Autodesk Inventor part; units mm, degrees
ref_plane "YZ Plane" through (0, 0, 0) normal (1, 0, 0) x (0, 1, 0)
ref_plane "XZ Plane" through (0, 0, 0) normal (0, 1, 0) x (-1, 0, 0)
ref_plane "XY Plane" through (0, 0, 0) normal (0, 0, 1) x (1, 0, 0)
sketch "Sketch1" plane through (0, 0, 0) normal (0, 1, 0) x (-1, 0, 0)
  arc A0 (9.525, 0) -> (0, -9.525) centre (0, 0) ccw
  line L0 (0, 0) -> (0, -696.722) construction
  arc A1 (0, -687.197) -> (9.525, -696.722) centre (0, -696.722) ccw
  line L1 (9.525, -696.722) -> (9.525, 0)
  line L2 (-9.525, 0) -> (-9.525, -696.722)
  circle A2 centre (0, -696.722) radius 4.7625
  circle A3 centre (0, 0) radius 4.7625
  dimension "d0" = 19.05
  dimension "d2" = 19.05
  dimension "d3" = 9.525
  dimension "d4" = 9.525
  dimension "d10" = 696.722
extrude "Extrusion2" add sketch "Sketch1" along normal blind 6.35
properties part number "steeringlinkage" material "Steel, Mild"
Source: CAD feature listing. Evaluate the final solid. Frame: model axes, mm. Coordinates: 2 decimals unless noted, no trailing zeros. Write each question's results on one line, items separated by ' | '. Start each with the question number.
1. Material intervals for L1, parallel to Z at x = 0.5, y = 4.5; L2, parallel to Z at x = 0, y = 3.5 (1 decimal); L3, parallel to Z at x = -5.75, y = 3.25, sorted ascending.
2. Pin query (flat end, axial travel): pin 1 (2 mm diameter, centred on x = 4.5, y = 5.5, fed in from +Z); pin 2 (5.5 mm diameter, centred on x = 0, z = 0, fed in from +Y) (3 decimals). Return the tip coordinate at first contact, or that it passes through.
3. Section A-A, the plane x = 0. State how many separate pieces and enclosed holes the cut face has, then the cut area to 3 significant figures.
Solution:
1) L1: -706.23 to -701.46, -691.99 to -4.74, 4.74 to 9.51 | L2: -706.2 to -701.5, -692 to -4.8, 4.8 to 9.5 | L3: -704.32 to 7.59
2) pin 1: z = 8.86 | pin 2: through
3) separate pieces: 3 | enclosed holes: 0 | area: 4,420 mm²
